The listing builds one solid part. Answer for the finished solid, in the listing's coordinates (mm). A direction names the side the tool comes from. Give positions to 0.01 mm unless a question says otherwise; leave off trailing zeros. Write each loop counter-clockwise with the first axis right and the second up, starting at its lowest first coordinate (ties: lowest second). Pieces come first, ordered by that corner, then holes. Notation, with made-up numbers: M 2.25,20 L 7.25,20 A23 cw 7.25,58 Z; hole C -37.75,8.5 d7. An arc over 180 degrees is marked long. Return JSON: item names as keys, results as strings.
from build123d import *

# Parameters (mm, degrees)
BOTTOM_SECTION_BASE_SKETCH_W             = 15
BOTTOM_SECTION_BASE_SKETCH_H             = 15
BOTTOM_SECTION_EXTRUDE_DEPTH             = 40
HINGE_CUTOUT_SKETCH_W                    = 7
HINGE_CUTOUT_SKETCH_H                    = 15
HINGE_CUTOUT_EXTRUDED_CUT_DEPTH          = 15
HINGE_HOLE_SKETCH_R                      = 1
HINGE_HOLE_EXTRUDED_CUT_DEPTH            = 44.373378932
HINGER_CORNER_FILLETS_R                  = 5
STYLE_FILLETS_R                          = 1
ROUTING_HOLES_SKETCH_W                   = 2
ROUTING_HOLES_SKETCH_H                   = 2
ROUTING_HOLES_EXTRUDED_CUT_DEPTH         = 42.382363393
BACKING_START                            = -3.5
BACKING_EXTRUDE_DEPTH                    = 7
BOTTOM_SECTION_CONNECTION_HOLE_R         = 1.75
BOTTOM_SECTION_CONNECTION_HOLE_CUT_DEPTH = 3
SKETCH2_W                                = 7
SKETCH2_H                                = 2
BOTTOM_EXTENSION_EXTRUDE_DEPTH           = 6.5
FILLET1_R                                = 0.5


# Read off the part's stored shape, not the designer's step: Backing Extrude
with BuildPart() as part:
    # Bottom Section Base Sketch → Bottom Section Extrude (new body)
    with BuildSketch(Plane.XY):
        Rectangle(BOTTOM_SECTION_BASE_SKETCH_W, BOTTOM_SECTION_BASE_SKETCH_H)
    extrude(amount=BOTTOM_SECTION_EXTRUDE_DEPTH)

    # Hinge Cutout Sketch → Hinge Cutout Extruded Cut (cut)
    with BuildSketch(Plane.XY):
        Rectangle(HINGE_CUTOUT_SKETCH_W, HINGE_CUTOUT_SKETCH_H)
    hinge_cutout_extruded_cut = extrude(amount=HINGE_CUTOUT_EXTRUDED_CUT_DEPTH, mode=Mode.SUBTRACT)

    # Hinge Hole Sketch → Hinge Hole Extruded Cut (cut, through all)
    with BuildSketch(Plane(origin=(7.5, 0, 0), x_dir=(0, 0, -1), z_dir=(1, 0, 0))):
        with Locations((-5, 0)):
            Circle(HINGE_HOLE_SKETCH_R)
    hinge_hole_extruded_cut = extrude(amount=-HINGE_HOLE_EXTRUDED_CUT_DEPTH, mode=Mode.SUBTRACT)

    # Hinge and Hole Cutout Mirror: Hinge Cutout Extruded Cut, Hinge Hole Extruded Cut across plane
    add(hinge_cutout_extruded_cut.mirror(Plane.XY.offset(20)), mode=Mode.SUBTRACT)
    add(hinge_hole_extruded_cut.mirror(Plane.XY.offset(20)), mode=Mode.SUBTRACT)

    # Hinger Corner Fillets
    hinger_corner_fillets_edges = [part.edges().sort_by_distance(p)[0] for p in [
        (5.5, -7.5, 0),
        (-5.5, 7.5, 0),
        (-5.5, -7.5, 40),
        (-5.5, 7.5, 40),
        (5.5, -7.5, 40),
        (-5.5, -7.5, 0),
        (5.5, 7.5, 0),
        (5.5, 7.5, 40),
    ]]
    fillet(hinger_corner_fillets_edges, radius=HINGER_CORNER_FILLETS_R)

    # Style Fillets
    style_fillets_edges = [part.edges().sort_by_distance(p)[0] for p in [
        (7.5, 0, 40),
        (7.5, 7.5, 20),
        (-7.5, 7.5, 20),
        (7.5, 0, 0),
        (7.5, -7.5, 20),
        (7.5, 6.035533906, 1.464466094),
        (7.5, -6.035533906, 1.464466094),
        (7.5, -6.035533906, 38.535533906),
        (7.5, 6.035533906, 38.535533906),
        (-7.5, -7.5, 20),
        (-7.5, 0, 40),
        (-7.5, 0, 0),
        (-7.5, -6.035533906, 1.464466094),
        (-7.5, 6.035533906, 1.464466094),
        (-7.5, 6.035533906, 38.535533906),
        (-7.5, -6.035533906, 38.535533906),
    ]]
    fillet(style_fillets_edges, radius=STYLE_FILLETS_R)

    # Routing Holes Sketch → Routing Holes Extruded Cut (cut, through all)
    with BuildSketch(Plane.XY):
        with Locations((0, 4.5)):
            Rectangle(ROUTING_HOLES_SKETCH_W, ROUTING_HOLES_SKETCH_H)
        with Locations((0, -4.5)):
            Rectangle(ROUTING_HOLES_SKETCH_W, ROUTING_HOLES_SKETCH_H)
    extrude(amount=ROUTING_HOLES_EXTRUDED_CUT_DEPTH, mode=Mode.SUBTRACT)

    # Backing Extrude outline → Backing Extrude (add)
    with BuildSketch(Plane.YZ.offset(BACKING_START)):
        Polygon((-7.5, 29.963646865), (-7.5, 25), (-5.5, 25), (-5.5, 29.973325422), align=None)
    extrude(amount=BACKING_EXTRUDE_DEPTH)

    # Bottom Section Connection Hole → Bottom Section Connection Hole Cut (cut)
    with BuildSketch(Plane(origin=(7.5, 0, 0), x_dir=(0, 0, -1), z_dir=(1, 0, 0))):
        with Locations((-20, 0)):
            Circle(BOTTOM_SECTION_CONNECTION_HOLE_R)
    bottom_section_connection_hole_cut = extrude(amount=-BOTTOM_SECTION_CONNECTION_HOLE_CUT_DEPTH, mode=Mode.SUBTRACT)

    # Sketch2 → Bottom extension Extrude (add)
    with BuildSketch(Plane(origin=(0, 0, 15), x_dir=(-1, 0, 0), z_dir=(0, 0, -1))):
        with Locations((0, -6.5)):
            Rectangle(SKETCH2_W, SKETCH2_H)
    extrude(amount=BOTTOM_EXTENSION_EXTRUDE_DEPTH)

    # Connection Hole Mirror: Bottom Section Connection Hole Cut across plane
    add(bottom_section_connection_hole_cut.mirror(Plane(origin=(0, 0, 0), x_dir=(0, 0, 1), z_dir=(1, 0, 0))), mode=Mode.SUBTRACT)

    # Fillet1
    fillet1_edges = [part.edges().sort_by_distance(p)[0] for p in [
        (-1, -4.5, 25),
        (0, -3.5, 25),
        (1, -4.5, 25),
        (0, 5.5, 25),
        (1, 4.5, 25),
        (0, 3.5, 25),
        (-1, 4.5, 25),
        (-1, 4.5, 15),
        (0, 3.5, 15),
        (1, 4.5, 15),
        (0, 5.5, 15),
        (1, -4.5, 15),
        (0, -3.5, 15),
        (-1, -4.5, 15),
    ]]
    fillet(fillet1_edges, radius=FILLET1_R)


solid = part.part
Item 1: A cutting plane is placed at D-D, the plane y = 0. Count the separate pieces of the cut face and the enclosed holes in it, plus the area to 3 significant figures.
Geometry results:
{"separate pieces": "5", "enclosed holes": "0", "area": "336 mm2"}
Item 2: Given pin 1 Ø1.6 at (y, z) = (0, 35) entering from -X; pin 2 Ø1 at (y, z) = (0.5, 19.5) entering from +X; pin 3 Ø3 at (y, z) = (0, 5) entering from -X; pin 4 Ø3.5 at (x, y) = (-0.5, 0) entering from +Z, each flat-ended and moving along its own axis, determine where each tip first touches the part or whether it passes through.
Geometry results:
{"pin 1": "passes through", "pin 2": "stops at x = 4.5", "pin 3": "stops at x = -7.5", "pin 4": "stops at z = 25"}
Item 3: A cutting plane is placed at A-A, the plane z = 7. Write down the section's boundary in (x, y).
Geometry results:
{"outline": "M -7.5,-6.5 A1 ccw -6.5,-7.5 L -3.5,-7.5 L -3.5,7.5 L -6.5,7.5 A1 ccw -7.5,6.5 Z; M 3.5,-7.5 L 6.5,-7.5 A1 ccw 7.5,-6.5 L 7.5,6.5 A1 ccw 6.5,7.5 L 3.5,7.5 Z"}
Item 4: Determine the mould class of faces 6 (the cylindrical face through (-4.98, -6.07, 38.5)), 7 (the flat face through (0, -6, 8.5)), 8 (the flat face through (3.5, 0, 33)), 9 (the flat face through (-7.5, -3, 20)) for opening direction X: +X half, -X half, draft (parallel to the pull), parting line (faces both ways), or undercut.
Geometry results:
{"face 6": "draft", "face 7": "undercut", "face 8": "undercut", "face 9": "-X half"}
Item 5: A cutting plane is placed at B-B, the plane z = 20. Write down the section's boundary in (x, y).
Geometry results:
{"outline": "M -7.5,-6.5 A1 ccw -6.5,-7.5 L 6.5,-7.5 A1 ccw 7.5,-6.5 L 7.5,-1.75 L 4.5,-1.75 L 4.5,1.75 L 7.5,1.75 L 7.5,6.5 A1 ccw 6.5,7.5 L -6.5,7.5 A1 ccw -7.5,6.5 L -7.5,1.75 L -4.5,1.75 L -4.5,-1.75 L -7.5,-1.75 Z; hole M -1,-5.5 L 1,-5.5 L 1,-3.5 L -1,-3.5 Z; hole M -1,3.5 L 1,3.5 L 1,5.5 L -1,5.5 Z"}
Item 6: Which of the six approach directions +Z, -Z, +X, -X, +Y, -Y give full straight-line access (tool end or side, diameter ignored) to faces 1 (the flat face through (-1, 4, 20)), 2 (the flat face through (-3.5, 0, 7)), 3 (the flat face through (5, 0, 40)), 4 (the flat face through (5, 0, 0)), 5 (the flat face through (-4.5, 0, 20))?
Geometry results:
{"face 1": "+Z, -Z", "face 2": "-Z, +Y", "face 3": "+Z, +X, -X, +Y, -Y", "face 4": "-Z, +X, -X, +Y, -Y", "face 5": "-X"}
Item 7: Find the intervals of material crossed by line 1 (X direction, y = 6.5, z = 9.5); line 2 (Y direction, x = 5.85, z = 20); line 3 (Z direction, x = 5.5, y = 0.5), in increasing order.
Geometry results:
{"line 1": "x = -7.5 to -3.5, 3.5 to 7.5", "line 2": "y = -7.5 to -1.75, 1.75 to 7.5", "line 3": "z = 0 to 4.13, 5.87 to 18.32, 21.68 to 34.13, 35.87 to 40"}
Item 8: A cutting plane is placed at C-C, the plane x = 5.25. Write down the section's boundary in (y, z), plus the area to 3 significant figures.
Geometry results:
{"outline": "M -7.5,5 A5 ccw -2.5,0 L 2.5,0 A5 ccw 7.5,5 L 7.5,35 A5 ccw 2.5,40 L -2.5,40 A5 ccw -7.5,35 Z; hole C 0,20 d3.5; hole C 0,5 d2; hole C 0,35 d2", "area": "563 mm2"}
